Build history of the part. All positions in model axes, mm. A direction names the side the tool comes from. Give positions to 0.01 mm unless a question says otherwise; leave off trailing zeros. Order: outer loops, then holes, each group sorted by start corner. A loop starts at its lowest first (then second) coordinate and runs counter-clockwise, first axis right, second up. Notation, with made-up numbers: (26.5, 48) - (68.5, 48) arc R17 cw to (68.5, 78) - close; hole circle Ø5 at (28, -30.75). An arc over 180 degrees is marked (long way). Answer in a Markdown table with one row per item.
Autodesk Inventor part; units mm, degrees
ref_plane "YZ Plane" through (0, 0, 0) normal (1, 0, 0) x (0, 1, 0)
ref_plane "XZ Plane" through (0, 0, 0) normal (0, 1, 0) x (-1, 0, 0)
ref_plane "XY Plane" through (0, 0, 0) normal (0, 0, 1) x (1, 0, 0)
sketch "Sketch1" plane through (0, 0, 0) normal (1, 0, 0) x (0, 1, 0)
  line L0 (0, 0) -> (241.3, 0)
  line L1 (241.3, 0) -> (241.3, -25.4)
  line L2 (241.3, -25.4) -> (0, -25.4)
  line L3 (0, -25.4) -> (0, 0)
  line L4 (6.3489, -9.0357) -> (12.6978, -5.3677)
  line L5 (12.6978, -5.3677) -> (19.0489, -9.0319)
  line L6 (19.0489, -9.0319) -> (19.0511, -16.3643)
  line L7 (19.0511, -16.3643) -> (12.7022, -20.0323)
  line L8 (12.7022, -20.0323) -> (6.3511, -16.3681)
  line L9 (6.3511, -16.3681) -> (6.3489, -9.0357)
  point P0 (12.7, -12.7)
  dimension "d0" = 241.3
  dimension "d1" = 25.4
  dimension "d3" = 12.7
  dimension "d4" = 12.7
extrude "Extrusion1" add sketch "Sketch1" along normal blind 25.4
sketch "Sketch2" plane through (0, 241.3, 0) normal (0, 1, 0) x (1, 0, 0)
  line L0 (0, 25.4) -> (25.4, 25.4)
  line L1 (0, 0) -> (25.4, 0)
  line L2 (25.4, 0) -> (25.4, 25.4)
  line L3 (25.4, 25.4) -> (0, 25.4)
  line L4 (0, 25.4) -> (0, 0)
  line L5 (22.225, 3.175) -> (3.175, 3.175)
  line L6 (3.175, 3.175) -> (3.175, 22.225)
  line L7 (3.175, 22.225) -> (22.225, 22.225)
  line L8 (22.225, 22.225) -> (22.225, 3.175)
  dimension "d7" = 3.175
extrude "Extrusion2" cut sketch "Sketch2" against normal blind 228.6 contours L5 L6 L7 L8
sketch "Sketch3" plane through (25.4, 0, 0) normal (1, 0, 0) x (0, 0, -1)
  line L0 (0, 241.3) -> (0, 190.5)
  line L1 (0, 0) -> (0, 241.3)
  line L2 (0, 241.3) -> (-3.175, 241.3)
  line L3 (-3.175, 241.3) -> (-3.175, 190.5)
  line L4 (-3.175, 190.5) -> (0, 190.5)
  line L5 (0, 190.5) -> (0, 241.3)
  arc A0 (-3.175, 241.3) -> (-46.143, 196.9282) centre (-8.4506, 203.4185) ccw
  line L6 (-3.175, 241.3) -> (-3.175, 238.125)
  arc A1 (-3.175, 238.125) -> (-42.9327, 197.9157) centre (-7.6224, 202.7623) ccw
  line L7 (-42.9327, 197.9157) -> (-46.143, 196.9282)
  dimension "d11" = 50.8
  dimension "d13" = 3.175
  dimension "d15" = 3.175
extrude "Extrusion3" add sketch "Sketch3" against normal blind 25.4 contours L0 L4 L3 L2
sketch "Sketch4" plane through (25.4, 0, 0) normal (1, 0, 0) x (0, 0, -1)
  point P0 (0, 0)
sketch "Sketch5" plane through (25.4, 0, 0) normal (1, 0, 0) x (0, 0, -1)
  line L0 (-3.175, 241.3) -> (-3.175, 190.5)
  line L1 (-3.175, 241.3) -> (-3.175, 196.85)
  line L2 (-3.175, 196.85) -> (-41.275, 196.85)
  arc A0 (-3.175, 241.3) -> (-41.275, 196.85) centre (-8.1247, 206.989) ccw
  line L3 (-41.275, 196.85) -> (-38.5091, 198.4089)
  line L4 (-3.175, 241.3) -> (-3.175, 238.125)
  arc A1 (-3.175, 238.125) -> (-38.5091, 198.4089) centre (-8.433, 207.227) ccw
  point P0 (0, 0)
  dimension "d18" = 44.45
  dimension "d19" = 38.1
  dimension "d20" = 3.175
  dimension "d21" = 3.175
extrude "Extrusion4" add sketch "Sketch5" against normal blind 25.4 contours L0 A1 L3 A0
sketch "Sketch6" plane through (25.4, 0, 0) normal (1, 0, 0) x (0, 0, -1)
  line L0 (0, 0) -> (25.4, 0)
  line L1 (25.4, 0) -> (25.4, 241.3)
  line L2 (12.7618, 20.0321) -> (19.0807, 16.3125)
  line L3 (19.0807, 16.3125) -> (19.0189, 8.9804)
  line L4 (19.0189, 8.9804) -> (12.6382, 5.3679)
  line L5 (12.6382, 5.3679) -> (6.3193, 9.0875)
  line L6 (6.3193, 9.0875) -> (6.3811, 16.4196)
  line L7 (6.3811, 16.4196) -> (12.7618, 20.0321)
  point P0 (12.7, 12.7)
  point P1 (12.7, 12.7)
  dimension "d25" = 12.7
  dimension "d26" = 12.7
  dimension "d27" = 12.7
extrude "Extrusion5" cut sketch "Sketch6" against normal blind 25.4
properties part number "claw"
1. Two-plate mould, pull along Z, no slides. Class faces 1 (the face through (13, 129, -22.225)), 2 (the face through (13, 122, -25.4)), 3 (the face through (13, 94, 0)): +Z half, -Z half, draft (parallel to the pull), parting line (faces both ways), or undercut.
Check result:
| item | result |
|---|---|
| face 1 | undercut |
| face 2 | -Z half |
| face 3 | +Z half |
2. Drop flat-ended pins along their axis: P1, Ø1.5, axis at x = 12, z = -10.5, coming from the +Y side; P2, Ø1.5, axis at x = 7.5, z = 5.5, coming from the +Y side; P3, Ø5.5, axis at x = 14, y = 130.5, coming from the +Z side. Give the stop position or say it passes through.
Check result:
| item | result |
|---|---|
| P1 | stops at y = 6.35 |
| P2 | stops at y = 241.6 |
| P3 | stops at z = 0 |
3. Which spindle directions (+Z, -Z, +X, -X, +Y, -Y) get a long thin tool onto all of the face, cutting with end or side? Do faces 4 (the face through (0, 130, -11)), 5 (the face through (12.88, 228.39, 31.55)), 6 (the face through (13, 241.3, -2)), 7 (the face through (13, 215, 3.175)), 8 (the face through (3.175, 129, -13)). Say none if no direction does.
Check result:
| item | result |
|---|---|
| face 4 | +Z, -Z, -X, +Y, -Y |
| face 5 | +X, -X |
| face 6 | -Z, +X, -X, +Y |
| face 7 | +X, -X, -Y |
| face 8 | +Y |
4. Cut at C-C on z = 27.5. Write the cut outline in (x, y), and give its area (3 significant figures).
Check result:
| item | result |
|---|---|
| outline | (0, 232.1) - (25.4, 232.1) - (25.4, 235.74) - (0, 235.74) - close |
| area | 92.3 mm² |
5. Probe line 1 (Z direction, x = 8, y = 190) (3 decimals); line 2 (X direction, y = 182.5, z = -11.5) (3 decimals); line 3 (Z direction, x = 17.5, y = 222.5) (3 decimals). List the from-to ranges inside material, lowest first.
Check result:
| item | result |
|---|---|
| line 1 | z = -25.4 to -22.225, -3.175 to 0 |
| line 2 | x = 0 to 3.175, 22.225 to 25.4 |
| line 3 | z = -25.4 to -22.225, -3.175 to 3.175, 35.802 to 39.127 |
6. Cut at A-A on y = 129. Write the cut outline in (x, z) (3 decimals).
Check result:
| item | result |
|---|---|
| outline | (0, -25.4) - (25.4, -25.4) - (25.4, 0) - (0, 0) - close; hole (3.175, -22.225) - (22.225, -22.225) - (22.225, -3.175) - (3.175, -3.175) - close |
